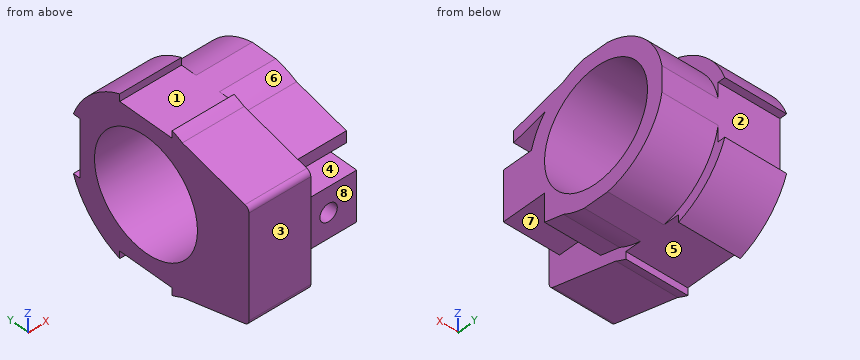
```python
from build123d import *

# Parameters (mm, degrees)
CROQUIS1_R              = 10
SALIENTE_EXTRUIR1_DEPTH = 11
CROQUIS2_R              = 10
SALIENTE_EXTRUIR2_DEPTH = 10
CORTAR_EXTRUIR3_START   = -10
CORTAR_EXTRUIR3_DEPTH   = 10
CROQUIS8_R              = 1.55
CORTAR_EXTRUIR4_DEPTH   = 5
CORTAR_EXTRUIR5_REACH   = 52.656


with BuildPart() as part:
    # Croquis1 → Saliente-Extruir1 (new body)
    with BuildSketch(Plane(origin=(0, 0, 0), x_dir=(0, 0, -1), z_dir=(1, 0, 0))):
        with BuildLine():
            Line((-5.780776406, 0), (-24.219223594, 0))
            ThreePointArc((-24.219223594, 0), (-24.834635803, 0.211794562), (-25.189366094, 0.757464375))
            Line((-25.189366094, 0.757464375), (-28.235294118, 12.941176471))
            ThreePointArc((-28.235294118, 12.941176471), (-15, 35), (-1.764705882, 12.941176471))
            Line((-1.764705882, 12.941176471), (-4.810633906, 0.757464375))
            ThreePointArc((-4.810633906, 0.757464375), (-5.165364197, 0.211794562), (-5.780776406, 0))
        make_face()
        with Locations((-15, 20)):
            Circle(CROQUIS1_R, mode=Mode.SUBTRACT)
    extrude(amount=SALIENTE_EXTRUIR1_DEPTH)

    # Croquis2 → Saliente-Extruir2 (add)
    with BuildSketch(Plane(origin=(11, 0, 0), x_dir=(0, 0, -1), z_dir=(1, 0, 0))):
        with BuildLine():
            Line((-23.438447187, 2), (-6.561552813, 2))
            Line((-6.561552813, 2), (-3.643105675, 13.673788552))
            ThreePointArc((-3.643105675, 13.673788552), (-15, 33), (-26.356894325, 13.673788552))
            Line((-26.356894325, 13.673788552), (-23.438447187, 2))
        make_face()
        with Locations((-15, 20)):
            Circle(CROQUIS2_R, mode=Mode.SUBTRACT)
    extrude(amount=SALIENTE_EXTRUIR2_DEPTH)

    # Croquis3 → Cortar-Extruir3 (cut)
    with BuildSketch(Plane(origin=(21, 0, 0), x_dir=(0, 0, -1), z_dir=(1, 0, 0)).offset(CORTAR_EXTRUIR3_START)):
        Polygon((-9.561552813, 2), (-9.561552813, 10), (-4.561552813, 10), (-6.561552813, 2), align=None)
        with BuildLine():
            Line((-23.438447187, 2), (-18.438447187, 2))
            Line((-18.438447187, 2), (-18.438447187, 6.945227656))
            Line((-18.438447187, 6.945227656), (-18.438447187, 7.462971606))
            ThreePointArc((-18.438447187, 7.462971606), (-21.059353424, 8.498511571), (-23.395524099, 10.074518898))
            Line((-23.395524099, 10.074518898), (-23.194590952, 9.270786312))
            Line((-23.194590952, 9.270786312), (-21.876894374, 4))
            Line((-21.876894374, 4), (-23.938447187, 4))
            Line((-23.938447187, 4), (-23.438447187, 2))
        make_face()
    extrude(amount=CORTAR_EXTRUIR3_DEPTH, mode=Mode.SUBTRACT)

    # Croquis8 → Cortar-Extruir4 (cut)
    with BuildSketch(Plane.XZ.offset(-2)):
        with Locations(Location((16, 14, 0), (0, 0, 270))):
            Circle(CROQUIS8_R)
    extrude(amount=-CORTAR_EXTRUIR4_DEPTH, mode=Mode.SUBTRACT)

    # Croquis9 → Cortar-Extruir5 (cut, up to next)
    with BuildSketch(Plane.ZY, mode=Mode.PRIVATE) as cortar_extruir5_sk1:
        with BuildLine():
            Line((2.2, 20), (2.2, 25.1))
            Line((2.2, 25.1), (0.893618465, 25.1))
            ThreePointArc((0.893618465, 25.1), (0, 20), (0.893618465, 14.9))
            Line((0.893618465, 14.9), (2.2, 14.9))
            Line((2.2, 14.9), (2.2, 20))
        make_face()
    cortar_extruir5_tool1 = extrude(cortar_extruir5_sk1.sketch, amount=-CORTAR_EXTRUIR5_REACH, mode=Mode.PRIVATE) & part.part
    # Croquis9 → Cortar-Extruir5 (cut, up to next)
    with BuildSketch(Plane.ZY, mode=Mode.PRIVATE) as cortar_extruir5_sk2:
        with BuildLine():
            Line((15, 32.8), (20.1, 32.8))
            Line((20.1, 32.8), (20.1, 34.106381535))
            ThreePointArc((20.1, 34.106381535), (15, 35), (9.9, 34.106381535))
            Line((9.9, 34.106381535), (9.9, 32.8))
            Line((9.9, 32.8), (15, 32.8))
        make_face()
    cortar_extruir5_tool2 = extrude(cortar_extruir5_sk2.sketch, amount=-CORTAR_EXTRUIR5_REACH, mode=Mode.PRIVATE) & part.part
    # Croquis9 → Cortar-Extruir5 (cut, up to next)
    with BuildSketch(Plane.ZY, mode=Mode.PRIVATE) as cortar_extruir5_sk3:
        with BuildLine():
            Line((27.8, 14.9), (29.106381535, 14.9))
            ThreePointArc((29.106381535, 14.9), (30, 20), (29.106381535, 25.1))
            Line((29.106381535, 25.1), (27.8, 25.1))
            Line((27.8, 25.1), (27.8, 20))
            Line((27.8, 20), (27.8, 14.9))
        make_face()
    cortar_extruir5_tool3 = extrude(cortar_extruir5_sk3.sketch, amount=-CORTAR_EXTRUIR5_REACH, mode=Mode.PRIVATE) & part.part
    add(cortar_extruir5_tool1.solids().sort_by_distance((0, 20, 1.228659))[0], mode=Mode.SUBTRACT)
    add(cortar_extruir5_tool2.solids().sort_by_distance((0, 33.771341, 15))[0], mode=Mode.SUBTRACT)
    add(cortar_extruir5_tool3.solids().sort_by_distance((0, 20, 28.771341))[0], mode=Mode.SUBTRACT)


solid = part.part
```
The listing builds one solid part. Answer for the finished solid, in the listing's coordinates (mm). Face numbers are marked on the shaded views. A direction names the side the tool comes from. Coordinates: 2 decimals unless noted, no trailing zeros. Write each loop counter-clockwise with the first axis right and the second up, starting at its lowest first coordinate (ties: lowest second). Pieces come first, ordered by that corner, then holes. Notation, with made-up numbers: M 89.25,-7 L 111.25,-7 A31 ccw 111.25,21 Z; hole C -4.5,1.5 d3. An arc over 180 degrees is marked long. Use a Markdown table: item, result. Add a question column.
1. Section B-B (x = 10) is taken. Give the vertices of the cut face in (y, z).
2. Section D-D (x = 16) is taken. Give the vertices of the cut face in (y, z), plus the area to 3 significant figures.
3. For a pull along Z with two mould halves and no side action, classify the marked faces 1, 2, 3 and 4 as +Z half, -Z half, draft (parallel to the pull), parting line (faces both ways), or undercut.
4. Straight lines are drawn through the part: line 1 along X through (y, z) = (4.15, 14); line 2 along Y through (x, z) = (1.5, 15); line 3 along X through (y, z) = (25.5, 27.25). For each, find the intervals that lie inside material, in ascending order. Write a range as [from, to].
5. Section A-A (y = 20) is taken. Give the vertices of the cut face in (x, z), plus the area to 3 significant figures.
6. Section C-C (z = 13.5) is taken. Give the vertices of the cut face in (x, y).
7. Which of the six approach directions +Z, -Z, +X, -X, +Y, -Y give full straight-line access (tool end or side, diameter ignored) to the marked faces 5, 6, 7 and 8?
8. Given P1, Ø3, axis at y = 18, z = 5.5, coming from the +X side; P2, Ø5, axis at x = 14.5, z = 22.5, coming from the +Y side; P3, Ø9, axis at x = 17.5, y = 7.5, coming from the -Z side; P4, Ø3.5, axis at x = 16, z = 14, coming from the -Y side, each flat-ended and moving along its own axis, determine where each tip first touches the part or whether it passes through.
Data:
| question | item | result |
|---|---|---|
| 1 | outline | M 0,5.78 A1 ccw 0.76,4.81 L 12.94,1.76 A15 ccw 14.9,0.89 L 14.9,2.2 L 25.1,2.2 L 25.1,0.89 A15 ccw 34.11,9.9 L 32.8,9.9 L 32.8,20.1 L 34.11,20.1 A15 ccw 25.1,29.11 L 25.1,27.8 L 14.9,27.8 L 14.9,29.11 A15 ccw 12.94,28.24 L 0.76,25.19 A1 ccw 0,24.22 Z; hole C 20,15 d20 |
| 2 | outline | M 2,9.56 L 10,9.56 L 10,4.56 L 13.67,3.64 A13 ccw 17.73,2.2 L 22.27,2.2 A13 ccw 32.8,12.73 L 32.8,17.27 A13 ccw 22.27,27.8 L 17.73,27.8 A13 ccw 13.67,26.36 L 4,23.94 L 4,21.88 L 10.07,23.4 A13 ccw 7.46,18.44 L 2,18.44 L 2,15.55 L 7,15.55 L 7,12.45 L 2,12.45 Z; hole C 20,15 d20 |
| 2 | area | 262 mm2 |
| 3 | face 1 | +Z half |
| 3 | face 2 | undercut |
| 3 | face 3 | draft |
| 3 | face 4 | undercut |
| 4 | line 1 | x = [0, 14.45], [17.55, 21] |
| 4 | line 2 | y = [0, 10], [30, 32.8] |
| 4 | line 3 | x = [0, 11] |
| 5 | outline | M 0,2.2 L 21,2.2 L 21,5 L 0,5 Z; M 0,25 L 21,25 L 21,27.8 L 0,27.8 Z |
| 5 | area | 118 mm2 |
| 6 | outline | M 0,0 L 11,0 L 11,2 L 14.53,2 L 14.53,7 L 17.47,7 L 17.47,2 L 21,2 L 21,10.11 L 0,10.11 Z; M 0,29.89 L 21,29.89 L 21,32.8 L 0,32.8 Z |
| 7 | face 5 | -Z, +X, -X |
| 7 | face 6 | +Z, +X, -Y |
| 7 | face 7 | -Z, +X, -Y |
| 7 | face 8 | +Z, -Z, +X, -Y |
| 8 | P1 | stops at x = 21 |
| 8 | P2 | stops at y = 32 |
| 8 | P3 | stops at z = 4.06 |
| 8 | P4 | stops at y = 2 |
